from build123d import *

# Parameters (mm, degrees)
F0_R     = 25.4
F0_R_2   = 7.1501
F1_DEPTH = 76.2
F3_R     = 25.4
F3_R_2   = 7.1501
F4_DEPTH = 76.2


with BuildPart() as f1:
    # F0 (on Right) → F1 (new body)
    with BuildSketch(Plane.YZ):
        Circle(F0_R)
        Circle(F0_R_2, mode=Mode.SUBTRACT)
    extrude(amount=F1_DEPTH)


with BuildPart() as f4:
    # F3 (on Front) → F4 (new body)
    with BuildSketch(Plane.XZ):
        Circle(F3_R)
        Circle(F3_R_2, mode=Mode.SUBTRACT)
    extrude(amount=F4_DEPTH)


solid = f4.part
Can you work these out from the model? Positions are in its coordinate system, mm. Give positions to 0.01 mm unless a question says otherwise; leave off trailing zeros. Loops run counter-clockwise (first coordinate to the right, second up) from the corner with the lowest first, then second, coordinate; pieces in that order, holes last. Notation, with made-up numbers: (14, 67.25) - (48, 67.25) arc R30 cw to (48, 89.25) - close; hole circle Ø11 at (27, 88). An arc over 180 degrees is marked (long way). One line per item, written item: value.
(1) If we section it at A-A, the plane z = 0: List the corners of the cut face in (x, y) for me, plus the area to 3 significant figures.
Verdict:
outline: (-25.4, -76.2) - (-7.15, -76.2) - (-7.15, 0) - (-25.4, 0) - close; (7.15, -76.2) - (25.4, -76.2) - (25.4, 0) - (7.15, 0) - close
area: 2,780 mm^2
(2) If we section it at C-C, the plane y = -71: List the corners of the cut face in (x, z) for me, plus the area to 3 significant figures.
Verdict:
outline: circle Ø50.8 at (0, 0); hole circle Ø14.3 at (0, 0)
area: 1,870 mm^2
(3) If we mould it in two halves opening along Z, with no side actions, what happens to faces 1 (the face through (5.3, -76.2, -5.3)), 2 (the face through (-1.55, -37.57, -6.98)), 3 (the face through (-5.506, -37.567, -24.796))? For each: released by +Z, released by -Z, zero draft, split by the parting line, or undercut.
Verdict:
face 1: zero draft
face 2: undercut
face 3: split by the parting line
(4) I need wall thicknesses on line 1 along Z through (x, y) = (0, -52.5); line 2 along X through (y, z) = (-66, 2); line 3 along X through (y, z) = (-48, -4). Which ranges of each line are inside material? Lowest first, please.
Verdict:
line 1: -25.4 to -7.15, 7.15 to 25.4
line 2: -25.32 to -6.86, 6.86 to 25.32
line 3: -25.08 to -5.93, 5.93 to 25.08
(5) If we section it at D-D, the plane x = -12: List the corners of the cut face in (y, z) for me, plus the area to 3 significant figures.
Verdict:
outline: (-76.2, -22.39) - (0, -22.39) - (0, 22.39) - (-76.2, 22.39) - close
area: 3,410 mm^2
(6) If we section it at B-B, the plane x = 0: List the corners of the cut face in (y, z) for me, plus the area to 3 significant figures.
Verdict:
outline: (-76.2, -25.4) - (0, -25.4) - (0, -7.15) - (-76.2, -7.15) - close; (-76.2, 7.15) - (0, 7.15) - (0, 25.4) - (-76.2, 25.4) - close
area: 2,780 mm^2
(7) I'm going to push flat-ended pins straight in: pin 1 (10 mm diameter, centred on x = -4.5, y = -25.5, fed in from -Z); pin 2 (4 mm diameter, centred on y = -35.5, z = -6, fed in from +X); pin 3 (2 mm diameter, centred on x = -4.5, y = -21.5, fed in from -Z). Where does each tip first touch, or does it pass through?
Verdict:
pin 1: z = -25.4
pin 2: x = 25.08
pin 3: z = -25.16
